Input: part model. Units: mm. Frame: model coordinates. A direction names the side the tool comes from. Give positions to 0.01 mm unless a question says otherwise; leave off trailing zeros. Loops run counter-clockwise (first coordinate to the right, second up) from the corner with the lowest first, then second, coordinate; pieces in that order, holes last. Notation, with made-up numbers: (-32, -32.5) -> (19, -32.5) arc R31 ccw to (19, -6.5) -> close; hole circle Ø10 at (-22, 77). An arc over 180 degrees is marked (long way). Answer as a JSON object with one key per item and string values.
```python
from build123d import *

# Parameters (mm, degrees)
F0_R     = 50.8
F1_DEPTH = 63.5
F3_DEPTH = 76.2
F5_DEPTH = 76.2


with BuildPart() as f1:
    # F0 (on Top) → F1 (new body, symmetric)
    with BuildSketch(Plane.XY):
        Circle(F0_R)
    extrude(amount=F1_DEPTH, both=True)

    # F2 (on Front) → F3 (intersect, symmetric)
    with BuildSketch(Plane.XZ):
        Polygon((-9.978701, -39.75891), (21.740365, -4.641373), (14.060883, 42.053018), (-27.234341, 65.162434), (-71.04916, 47.285013), (-84.390123, 1.882818), (-57.211212, -36.855372), align=None)
    extrude(amount=F3_DEPTH, both=True, mode=Mode.INTERSECT)

    # F4 (on Right) → F5 (cut, symmetric)
    with BuildSketch(Plane.YZ):
        Polygon((-38.51945, 51.898345), (-59.98449, 15.143144), (-67.335531, -16.613351), (2.058293, -34.255847), (24.993537, 6.615937), align=None)
    extrude(amount=F5_DEPTH, both=True, mode=Mode.SUBTRACT)


solid = f1.part
```
Q1. Draft query along Y for faces 1 (the flat face through (-14.96, -6.32, 28.94)), 2 (the flat face through (2.13, 10.58, -26.35)), 3 (the flat face through (-22.057, 13.365, -14.106)), 4 (the cylindrical face through (-43.88, 25.6, 12.59)). Return one class per face: +Y half, -Y half, draft (parallel to the pull), parting line (faces both ways), or undercut.
Evaluation:
{"face 1": "undercut", "face 2": "draft", "face 3": "undercut", "face 4": "parting line"}
Q2. Access query for faces 5 (the flat face through (-8.601, -44.574, 41.531)), 6 (the flat face through (-28, 1, 63.5)). Directions: +Z, -Z, +X, -X, +Y, -Y. A direction counts if a zero-diameter tool reaches every point of the face in a straight line with its end or side. Return the directions, or none.
Evaluation:
{"face 5": "+X, -X", "face 6": "+Z, +X, -X, +Y, -Y"}
Q3. Section B-B, the plane x = 10.5. Return the cut outline in (y, z).
Evaluation:
{"outline": "(-49.7, 32.75) -> (-43.11, 44.05) -> (-49.7, 44.05) -> close; (-27.51, 44.05) -> (24.99, 6.62) -> (11.69, -17.09) -> (49.7, -17.09) -> (49.7, 44.05) -> close"}
Q4. Section A-A, the plane y = -41.5. Return the cut outline in (x, z).
Evaluation:
{"outline": "(-29.3, -38.57) -> (-9.98, -39.76) -> (4.99, -23.18) -> (-29.3, -23.18) -> close; (-29.3, 46.79) -> (5.59, 46.79) -> (-24.26, 63.5) -> (-29.3, 63.5) -> close"}
Q5. Pin query (flat end, axial travel): pin 1 (3 mm diameter, centred on y = 26, z = -13, fed in from -X); pin 2 (10 mm diameter, centred on x = 3, y = 15, fed in from -Z); pin 3 (8 mm diameter, centred on y = -5, z = 29, fed in from -X). Return the tip coordinate at first contact, or that it passes through.
Evaluation:
{"pin 1": "stops at x = -44.5", "pin 2": "stops at z = -30.93", "pin 3": "stops at x = -50.79"}
Q6. Section C-C, the plane x = 0. Return the cut outline in (y, z), then the cut area to 3 significant figures.
Evaluation:
{"outline": "(-50.8, -28.71) -> (-19.75, -28.71) -> (-50.8, -20.82) -> close; (-50.8, 30.87) -> (-39.67, 49.92) -> (-50.8, 49.92) -> close; (-35.75, 49.92) -> (24.99, 6.62) -> (5.17, -28.71) -> (50.8, -28.71) -> (50.8, 49.92) -> close", "area": "3,920 mm2"}
Q7. Ray query, line 1 along Z through (x, y) = (-12, -30); line 2 along Z through (x, y) = (-5.5, 14); line 3 along Y through (x, z) = (-45, -20.5). Return the intervals inside material, ascending.
Evaluation:
{"line 1": "z = -39.63 to -26.11, 45.82 to 56.64", "line 2": "z = -34.8 to -12.98, 14.45 to 53", "line 3": "y = 9.78 to 23.57"}
Q8. Section D-D, the plane z = -32.5. Return the cut outline in (x, y).
Evaluation:
{"outline": "(-50.71, 3.04) -> (-3.42, 3.04) -> (-3.42, 50.68) arc R50.8 ccw to start; (-50.57, -4.85) arc R50.8 ccw to (-3.42, -50.68) -> (-3.42, -4.85) -> close"}
